For this review, take the finished solid that the model builds, in its own axes (mm). Face numbers are marked on the shaded views. A direction names the side the tool comes from. Coordinates: 2 decimals unless noted, no trailing zeros. Order: outer loops, then holes, each group sorted by start corner. A loop starts at its lowest first (then second) coordinate and runs counter-clockwise, first axis right, second up.
from build123d import *

# Parameters (mm, degrees)
F0_R     = 10
F1_DEPTH = 54
F2_R     = 6
F3_DEPTH = 15
F4_R     = 18
F5_DEPTH = 75
F6_SIZE  = 2
F7_SIZE  = 1


with BuildPart() as f1:
    # F0 (on Front) → F1 (new body)
    with BuildSketch(Plane.XZ):
        Circle(F0_R)
    extrude(amount=F1_DEPTH)

    # F2 (on face) → F3 (join)
    with BuildSketch(Plane.XZ.offset(54)):
        Circle(F2_R)
    extrude(amount=F3_DEPTH)

    # F4 (on face) → F5 (join)
    with BuildSketch(Plane(origin=(0, 0, 0), x_dir=(-1, 0, 0), z_dir=(0, 1, 0))):
        Circle(F4_R)
    extrude(amount=F5_DEPTH)

    # F6
    f6_edges = [f1.edges().sort_by_distance(p)[0] for p in [
        (18, 75, 0),
    ]]
    chamfer(f6_edges, length=F6_SIZE)

    # F7
    f7_edges = [f1.edges().sort_by_distance(p)[0] for p in [
        (-6, -69, 0),
    ]]
    chamfer(f7_edges, length=F7_SIZE)


solid = f1.part
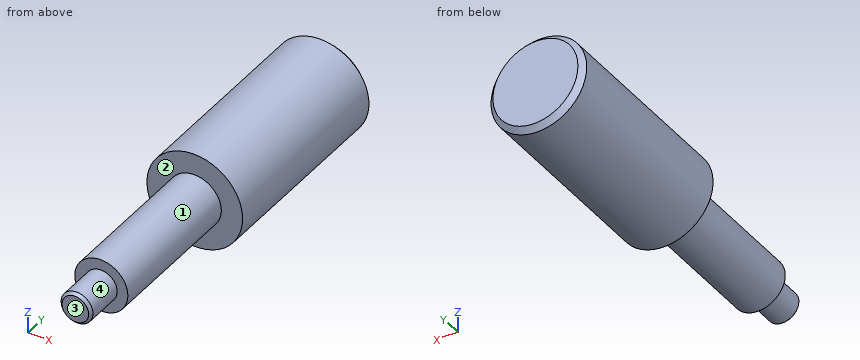
1. Machinability: for the marked faces 3 and 4, which of the approach directions +Z, -Z, +X, -X, +Y, -Y give a long, thin tool a straight path to every point of the face, cutting with its end or side? Answer none if there is none.
Answer below:
face 3: +Z, -Z, +X, -X, -Y
face 4: -Y
2. The part is to be moulded in two halves that separate along Z. For the marked faces 1 and 2, say which applies: +Z half, -Z half, draft (parallel to the pull), parting line (faces both ways), or undercut.
Answer below:
face 1: parting line
face 2: draft
3. Take a section at A-A, the plane z = 0. Give the boundary of the cut face in (x, y).
Answer below:
outline: (-18, 0) - (-10, 0) - (-10, -54) - (-6, -54) - (-6, -68) - (-5, -69) - (5, -69) - (6, -68) - (6, -54) - (10, -54) - (10, 0) - (18, 0) - (18, 73) - (16, 75) - (-16, 75) - (-18, 73) - close
4. Take a section at C-C, the plane y = 26.5. Give the boundary of the cut face in (x, z).
Answer below:
outline: circle Ø36 at (0, 0)
5. Clearance check with flat-ended pins moving along their axes: pin 1 Ø12 at (x, y) = (-11, -10.5) entering from +Z; pin 2 Ø4 at (y, z) = (26, 6) entering from -X; pin 3 Ø6 at (y, z) = (-12.5, 12) entering from +X. State where each tip first meets the part, or that it passes through.
Answer below:
pin 1: stops at z = 8.66
pin 2: stops at x = -17.55
pin 3: stops at x = 4.36
6. Take a section at B-B, the plane x = 0. Give the boundary of the cut face in (y, z).
Answer below:
outline: (-69, -5) - (-68, -6) - (-54, -6) - (-54, -10) - (0, -10) - (0, -18) - (73, -18) - (75, -16) - (75, 16) - (73, 18) - (0, 18) - (0, 10) - (-54, 10) - (-54, 6) - (-68, 6) - (-69, 5) - close
7. To check wall thickness, follow L1, parallel to Y at x = 5, z = -11; L2, parallel to Z at x = -1, y = 4; L3, parallel to Y at x = -6, z = -5.5. State the ranges of each line that lie inside material, in increasing order.
Answer below:
L1: y = 0 to 75
L2: z = -17.97 to 17.97
L3: y = -54 to 75
8. Take a section at D-D, the plane y = -8. Give the boundary of the cut face in (x, z).
Answer below:
outline: circle Ø20 at (0, 0)
